from build123d import *

# Parameters (mm, degrees)
EXTRUDE_1_DEPTH     = 30
SKETCH_3_W          = 5
SKETCH_3_H          = 20
CUT_EXTRUDE_1_DEPTH = 76.206382708
SKETCH_4_R          = 8
CUT_EXTRUDE_2_DEPTH = 78.717436911


with BuildPart() as part:
    # Эскиз1 → Бобышка-Вытянуть1 (new body)
    with BuildSketch(Plane.XY):
        Polygon((0, 0), (0, 8), (11, 8), (11, 28), (55, 28), (55, 8), (66, 8), (66, 0), (48, 0), (48, 20), (18, 20), (18, 0), align=None)
    extrude(amount=EXTRUDE_1_DEPTH)

    # Эскиз3 → Вырез-Вытянуть1 (cut, through all)
    with BuildSketch(Plane(origin=(0, 8, 0), x_dir=(1, 0, 0), z_dir=(0, 1, 0))):
        with Locations((2.5, -15)):
            Rectangle(SKETCH_3_W, SKETCH_3_H)
        with Locations((63.5, -15)):
            Rectangle(SKETCH_3_W, SKETCH_3_H)
    extrude(amount=-CUT_EXTRUDE_1_DEPTH, mode=Mode.SUBTRACT)

    # Эскиз4 → Вырез-Вытянуть2 (cut, through all)
    with BuildSketch(Plane(origin=(0, 28, 0), x_dir=(1, 0, 0), z_dir=(0, 1, 0))):
        with Locations(Location((33, -15, 0), (0, 0, 270))):
            Circle(SKETCH_4_R)
    extrude(amount=-CUT_EXTRUDE_2_DEPTH, mode=Mode.SUBTRACT)


solid = part.part
The listing builds one solid part. Answer for the finished solid, in the listing's coordinates (mm). A direction names the side the tool comes from. Coordinates: 2 decimals unless noted, no trailing zeros. Loops run counter-clockwise (first coordinate to the right, second up) from the corner with the lowest first, then second, coordinate; pieces in that order, holes last. Notation, with made-up numbers: (-6.75, -31.5) -> (25.25, -31.5) arc R16 cw to (25.25, -13.5) -> close; hole circle Ø1 at (63, -3). An arc over 180 degrees is marked (long way). Answer in a Markdown table with one row per item. Add a question column.
1. The part is cut by section A-A, the plane z = 15. Write down the section's boundary in (x, y), then the cut area to 3 significant figures.
2. The part is cut by section C-C, the plane y = 15.75. Write down the section's boundary in (x, z).
3. The part is cut by section D-D, the plane z = 27.75. Write down the section's boundary in (x, y).
4. For faces 3 (the flat face through (40, 20, 21)), 4 (the flat face through (61, 4, 15)), 5 (the flat face through (11, 18, 15)), determine the directions among +Z, -Z, +X, -X, +Y, -Y from which every point of the face is accessible in a straight line to the end or side of a thin tool.
5. Determine the mould class of faces 1 (the flat face through (5, 4, 15)), 2 (the flat face through (0, 4, 27)) for opening direction Z: +Z half, -Z half, draft (parallel to the pull), parting line (faces both ways), or undercut.
6. Consider line 1 (X direction, y = 26.25, z = 15); line 2 (X direction, y = 18.25, z = 1.75); line 3 (Y direction, x = 47.5, z = 7.5). Determine where each line is inside the solid, lowest interval first. Write a range as [from, to].
7. Flat-ended cylindrical pins translate along their axes: P1, Ø12, axis at y = 10, z = 19, coming from the +X side; P2, Ø9, axis at x = 3, z = 18.5, coming from the +Y side; P3, Ø4, axis at y = 5.5, z = 17.5, coming from the -X side. Find the tip coordinate at first contact, or state that the pin passes through.
8. The part is cut by section B-B, the plane x = 33. Write down the section's boundary in (y, z).
Answer below:
| question | item | result |
|---|---|---|
| 1 | outline | (5, 0) -> (18, 0) -> (18, 20) -> (25, 20) -> (25, 28) -> (11, 28) -> (11, 8) -> (5, 8) -> close; (41, 20) -> (48, 20) -> (48, 0) -> (61, 0) -> (61, 8) -> (55, 8) -> (55, 28) -> (41, 28) -> close |
| 1 | area | 600 mm2 |
| 2 | outline | (11, 0) -> (18, 0) -> (18, 30) -> (11, 30) -> close; (48, 0) -> (55, 0) -> (55, 30) -> (48, 30) -> close |
| 3 | outline | (0, 0) -> (18, 0) -> (18, 20) -> (48, 20) -> (48, 0) -> (66, 0) -> (66, 8) -> (55, 8) -> (55, 28) -> (11, 28) -> (11, 8) -> (0, 8) -> close |
| 4 | face 3 | +Z, -Z, -Y |
| 4 | face 4 | +X, +Y, -Y |
| 4 | face 5 | +Z, -Z, -X, +Y |
| 5 | face 1 | undercut |
| 5 | face 2 | draft |
| 6 | line 1 | [11, 25], [41, 55] |
| 6 | line 2 | [11, 18], [48, 55] |
| 6 | line 3 | [20, 28] |
| 7 | P1 | x = 61 |
| 7 | P2 | y = 8 |
| 7 | P3 | x = 5 |
| 8 | outline | (20, 0) -> (28, 0) -> (28, 7) -> (20, 7) -> close; (20, 23) -> (28, 23) -> (28, 30) -> (20, 30) -> close |
